Autodesk Fusion 360 part; units mm, degrees
sketch "Skizze1" plane through (0, 0, 0) normal (0, 0, 1) x (1, 0, 0)
  line L0 (15, -3.25) -> (-15, -3.25)
  line L1 (-15, -3.25) -> (-15, 3.25)
  line L2 (-15, 3.25) -> (15, 3.25)
  line L3 (15, 3.25) -> (15, -3.25)
  line L4 (15, -3.25) -> (-15, 3.25) construction
  line L5 (-15, -3.25) -> (15, 3.25) construction
  line L6 (-21.7851, 0.25) -> (21, 0.25) construction
  line L7 (10, 7.6042) -> (10, -9) construction
  line L8 (1.5, 8) -> (1.5, -9) construction
  line L9 (-3.5, 3.25) -> (-3.5, -3.25)
  line L10 (-12.5, 3.25) -> (-12.5, -3.25)
  circle A0 centre (10, 0.25) radius 1.25
  circle A1 centre (1.5, 0.25) radius 1.25
  dimension "d1" = 6.5
  dimension "d2" = 30
  dimension "d3" = 3
  dimension "d4" = 5
  dimension "d5" = 8.5
  dimension "d6" = 9
  dimension "d7" = 2.5
  dimension "d8" = 2.5
  dimension "d9" = 2.5
extrude "Extrusion1" add sketch "Skizze1" along normal blind 9
extrude "Extrusion2" cut sketch "Skizze1" along normal blind 6.4 contours L0 L2 L9 L10
sketch "Skizze2" plane through (0, 0, 9) normal (0, 0, 1) x (-1, 0, 0)
  circle A0 centre (-10, -0.25) radius 1.25
  circle A1 centre (-1.5, -0.25) radius 1.25
  line L0 (-15, -3.25) -> (15, -3.25)
  line L1 (15, -3.25) -> (15, 3.25)
  line L2 (15, 3.25) -> (-15, 3.25)
  line L3 (-15, 3.25) -> (-15, -3.25)
  line L4 (15.9329, -0.25) -> (-19.3468, -0.25) construction
  line L5 (-10, -6.1266) -> (-10, 7.3493) construction
  line L6 (-1.5, 6.35) -> (-1.5, -4.2794) construction
  circle A2 centre (-1.5, -0.25) radius 2
  circle A3 centre (-10, -0.25) radius 2
  dimension "d14" = 0.25
  dimension "d15" = 10
  dimension "d16" = 8.5
  dimension "d17" = 4
  dimension "d18" = 4
extrude "Extrusion3" cut sketch "Skizze2" against normal blind 4 contours A2
extrude "Extrusion4" cut sketch "Skizze2" against normal blind 4 contours A3
The model under review builds one solid part; all positions refer to its coordinate system, in mm. A direction names the side the tool comes from. Coordinates: 2 decimals unless noted, no trailing zeros. Order: outer loops, then holes, each group sorted by start corner. A loop starts at its lowest first (then second) coordinate and runs counter-clockwise, first axis right, second up. Notation, with made-up numbers: (77.5, -3) -> (114.5, -3) arc R38 cw to (114.5, 35) -> close; hole circle Ø11 at (-13.5, 32.5). An arc over 180 degrees is marked (long way). Answer in a Markdown table with one row per item. Add a question column.
Item 1: Clearance check with a flat-ended pin moving along its axis: pin 1 (1.2 mm diameter, centred on x = 1.5, y = -0.5, fed in from +Z). State where the tip first meets the part, or that it passes through.
Item 2: We need section C-C on x = 10. Write out the cut boundary in (y, z), plus the area to 3 significant figures.
Item 3: To check wall thickness, follow probe 1 along X at (y, z) = (0.25, 6.1); probe 2 along X at (y, z) = (-3, 4.25); probe 3 along Y at (x, z) = (10, 3.05). State the ranges of each line that lie inside material, in increasing order.
Item 4: Mouldability with a two-part tool opening along Y and no side actions: class faces 1 (the flat face through (3, 3.25, 4)), 2 (the cylindrical face through (11.587, 1.467, 7.028)), 3 (the flat face through (15, 0, 4)), 4 (the cylindrical face through (1.934, 2.202, 7.028)) as +Y half, -Y half, draft (parallel to the pull), parting line (faces both ways), or undercut.
Item 5: We need section A-A on z = 1.75. Write out the cut boundary in (x, y), plus the area to 3 significant figures.
Item 6: Machinability: for faces 5 (the flat face through (-8, 0, 6.4)), 6 (the flat face through (9, -1, 5)), 7 (the flat face through (-14, 0, 0)), which of the approach directions +Z, -Z, +X, -X, +Y, -Y give a long, thin tool a straight path to every point of the face, cutting with its end or side? Answer none if there is none.
Item 7: We need section B-B on y = 0.25. Write out the cut boundary in (x, z).
Item 8: We need section D-D on z = 6. Write out the cut boundary in (x, y).
Final values:
| question | item | result |
|---|---|---|
| 1 | pin 1 | stops at z = 5 |
| 2 | outline | (-3.25, 0) -> (-1, 0) -> (-1, 5) -> (-1.75, 5) -> (-1.75, 9) -> (-3.25, 9) -> close; (1.5, 0) -> (3.25, 0) -> (3.25, 9) -> (2.25, 9) -> (2.25, 5) -> (1.5, 5) -> close |
| 2 | area | 30.0 mm2 |
| 3 | probe 1 | x = -15 to -12.5, -3.5 to -0.5, 3.5 to 8, 12 to 15 |
| 3 | probe 2 | x = -15 to -12.5, -3.5 to 15 |
| 3 | probe 3 | y = -3.25 to -1, 1.5 to 3.25 |
| 4 | face 1 | +Y half |
| 4 | face 2 | undercut |
| 4 | face 3 | draft |
| 4 | face 4 | undercut |
| 5 | outline | (-15, -3.25) -> (-12.5, -3.25) -> (-12.5, 3.25) -> (-15, 3.25) -> close; (-3.5, -3.25) -> (15, -3.25) -> (15, 3.25) -> (-3.5, 3.25) -> close; hole circle Ø2.5 at (1.5, 0.25); hole circle Ø2.5 at (10, 0.25) |
| 5 | area | 127 mm2 |
| 6 | face 5 | -Z, +Y, -Y |
| 6 | face 6 | +Z |
| 6 | face 7 | -Z, +X, -X, +Y, -Y |
| 7 | outline | (-15, 0) -> (-12.5, 0) -> (-12.5, 6.4) -> (-3.5, 6.4) -> (-3.5, 0) -> (0.25, 0) -> (0.25, 5) -> (-0.5, 5) -> (-0.5, 9) -> (-15, 9) -> close; (2.75, 0) -> (8.75, 0) -> (8.75, 5) -> (8, 5) -> (8, 9) -> (3.5, 9) -> (3.5, 5) -> (2.75, 5) -> close; (11.25, 0) -> (15, 0) -> (15, 9) -> (12, 9) -> (12, 5) -> (11.25, 5) -> close |
| 8 | outline | (-15, -3.25) -> (-12.5, -3.25) -> (-12.5, 3.25) -> (-15, 3.25) -> close; (-3.5, -3.25) -> (15, -3.25) -> (15, 3.25) -> (-3.5, 3.25) -> close; hole circle Ø4 at (1.5, 0.25); hole circle Ø4 at (10, 0.25) |
